Check sheet for the modelled part. Datum: model origin and axes. Units: mm. A direction names the side the tool comes from. Round coordinates to 2 decimals unless told otherwise and drop trailing zeros. Order: outer loops, then holes, each group sorted by start corner. A loop starts at its lowest first (then second) coordinate and runs counter-clockwise, first axis right, second up. Notation, with made-up numbers: M 49,47 L 68,47 A21 ccw 68,60 Z; hole C 76,50.5 d4. An arc over 180 degrees is marked long. One line per item, written item: value. Start each with the question number.
(1) Access from +Z, -Z, +X, -X, +Y, -Y to the whole of each face (thin tool, end or side, straight path). Record for faces 1 (the face through (6.35, 2, 13)), 2 (the face through (27.49, 1.57, -8.02)), 3 (the face through (15.89, 1.57, -23.79)).
(2) Cross-section at A-A, the plane x = 11. Enter the section's corners in (y, z) (3 decimals).
(3) Cross-section at C-C, the plane y = 0.6. Count the separate pieces of the cut face and the enclosed holes in it, and give its area (3 significant figures).
(4) Depth check by flat-ended pin: pin 1 Ø1.5 at (y, z) = (0.5, -19) entering from -X; pin 2 Ø1.6 at (y, z) = (2, 14.5) entering from +X. Enter the tip coordinate at first touch or a pass-through.
(5) Release check for a two-part mould opening along X. For faces 4 (the face through (17.342, 1.565, 22.794)), 5 (the face through (28.44, 1.57, 3.36)), 6 (the face through (0, 2, 17)) record: released by +X, released by -X, zero draft, split by the parting line, or undercut.
(6) Thickness scan on L1, parallel to Z at x = 27.5, y = 1.3; L2, parallel to X at y = 2.9, z = 8.5; L3, parallel to Z at x = 6.5, y = 1. Record the ranges inside material, lowest first.
from build123d import *

# Parameters (mm, degrees)
BOSS_EXTRUDE1_DEPTH = 3.175
CUT_EXTRUDE1_DEPTH  = 3.175
CIRPATTERN1_DEPTH   = 3.175
SKETCH3_R           = 1
CUT_EXTRUDE2_DEPTH  = 3.175


# Read off the part's stored shape, not the designer's step: CirPattern1
with BuildPart() as part:
    # Sketch1 → Boss-Extrude1 (new body)
    with BuildSketch(Plane(origin=(0, 0, 0), x_dir=(1, 0, 0), z_dir=(0, 1, 0))):
        with BuildLine():
            Line((0, 29.6545), (0, 6.35))
            ThreePointArc((0, 6.35), (-6.35, 0), (0, -6.35))
            Line((0, -6.35), (0, -29.6545))
            ThreePointArc((0, -29.6545), (29.6545, 0), (0, 29.6545))
        make_face()
        with BuildLine():
            Line((6.35, 22.422694313), (6.35, 3.666174209))
            Line((6.35, 3.666174209), (20.182289022, 11.65225))
            ThreePointArc((20.182289022, 11.65225), (14.317514025, 18.387727222), (6.35, 22.422694313))
        make_face(mode=Mode.SUBTRACT)
        with BuildLine():
            Line((6.35, 0), (21.581607168, -8.793972499))
            ThreePointArc((21.581607168, -8.793972499), (23.3045, 0), (21.581607168, 8.793972499))
            Line((21.581607168, 8.793972499), (6.35, 0))
        make_face(mode=Mode.SUBTRACT)
        with BuildLine():
            Line((6.35, -3.666174209), (20.182289022, -11.65225))
            ThreePointArc((20.182289022, -11.65225), (14.317514025, -18.387727222), (6.35, -22.422694313))
            Line((6.35, -22.422694313), (6.35, -3.666174209))
        make_face(mode=Mode.SUBTRACT)
    extrude(amount=BOSS_EXTRUDE1_DEPTH)

    # Sketch2 → Cut-Extrude1 (cut)
    with BuildSketch(Plane(origin=(0, 3.175, 0), x_dir=(1, 0, 0), z_dir=(0, 1, 0))):
        Polygon((2.009170374, 29.586358422), (2.730257833, 27.469749607), (4.711979869, 27.199976048), (5.972614446, 29.046811304), align=None)
    extrude(amount=-CUT_EXTRUDE1_DEPTH, mode=Mode.SUBTRACT)


with BuildPart() as body_2:
    # of the pieces the cut leaves, the one that is kept (cut_extrude1_keep)
    add(part.part.solids().sort_by_distance((0, 0, -29.6545))[0])

    # CirPattern1 outline → CirPattern1 (cut)
    with BuildSketch(Plane(origin=(0, 0, 0), x_dir=(1, 0, 0), z_dir=(0, 1, 0))):
        with BuildLine():
            ThreePointArc((11.643715218, 27.272940182), (9.777824138, 27.996134115), (7.867406851, 28.59183939))
            Line((7.867406851, 28.59183939), (8.152034339, 26.373960405))
            Line((8.152034339, 26.373960405), (10.040188522, 25.714510801))
            Line((10.040188522, 25.714510801), (11.643715218, 27.272940182))
        make_face()
        with BuildLine():
            ThreePointArc((0, -29.6545), (0.935371957, -29.639744425), (1.869813063, -29.595492382))
            Line((1.869813063, -29.595492382), (0.878621718, -27.591112249))
            Line((0.878621718, -27.591112249), (0, -27.587246726))
            Line((0, -27.587246726), (0, -29.6545))
        make_face()
        with BuildLine():
            ThreePointArc((3.809498846, -29.408792712), (5.784253675, -29.084906389), (7.732668198, -28.628573363))
            Line((7.732668198, -28.628573363), (6.361766185, -26.862043524))
            Line((6.361766185, -26.862043524), (4.400181509, -27.252153199))
            Line((4.400181509, -27.252153199), (3.809498846, -29.408792712))
        make_face()
        with BuildLine():
            ThreePointArc((9.596192288, -28.058910596), (11.466730783, -27.347823595), (13.285052137, -26.51220021))
            Line((13.285052137, -26.51220021), (11.589481982, -25.054447882))
            Line((11.589481982, -25.054447882), (9.745052057, -25.827803075))
            Line((9.745052057, -25.827803075), (9.596192288, -28.058910596))
        make_face()
        with BuildLine():
            ThreePointArc((14.997592941, -25.582446643), (16.688811877, -24.512709528), (18.304033384, -23.331346556))
            Line((18.304033384, -23.331346556), (16.35187323, -22.240901357))
            Line((16.35187323, -22.240901357), (14.698653008, -23.3664514))
            Line((14.698653008, -23.3664514), (14.997592941, -25.582446643))
        make_face()
        with BuildLine():
            ThreePointArc((19.796831377, -22.078832344), (21.240827314, -20.693395692), (22.588096877, -19.213725556))
            Line((22.588096877, -19.213725556), (20.457727108, -18.534369503))
            Line((20.457727108, -18.534369503), (19.062094358, -19.966922897))
            Line((19.062094358, -19.966922897), (19.796831377, -22.078832344))
        make_face()
        with BuildLine():
            ThreePointArc((23.801215338, -17.688739883), (24.940010987, -16.043229793), (25.965234936, -14.324662123))
            Line((25.965234936, -14.324662123), (23.742191157, -14.083671764))
            Line((23.742191157, -14.083671764), (22.660181358, -15.765710644))
            Line((22.660181358, -15.765710644), (23.801215338, -17.688739883))
        make_face()
        with BuildLine():
            ThreePointArc((26.849966443, -12.588434067), (27.637838485, -10.748918742), (28.299853474, -8.860455044))
            Line((28.299853474, -8.860455044), (26.073392205, -9.067506284))
            Line((26.073392205, -9.067506284), (25.348448689, -10.931495795))
            Line((25.348448689, -10.931495795), (26.849966443, -12.588434067))
        make_face()
        with BuildLine():
            ThreePointArc((28.820675533, -6.982695186), (29.22599044, -5.023032253), (29.498216176, -3.04049546))
            Line((29.498216176, -3.04049546), (27.357731153, -3.68727507))
            Line((27.357731153, -3.68727507), (27.018960831, -5.658374932))
            Line((27.018960831, -5.658374932), (28.820675533, -6.982695186))
        make_face()
        with BuildLine():
            ThreePointArc((29.634217474, -1.096596968), (29.640701614, 0.904531949), (29.512208073, 2.901541813))
            Line((29.512208073, 2.901541813), (27.543641034, 1.841002417))
            Line((27.543641034, 1.841002417), (27.604645734, -0.158066973))
            Line((27.604645734, -0.158066973), (29.634217474, -1.096596968))
        make_face()
        with BuildLine():
            ThreePointArc((29.257928078, 4.833530266), (28.865321108, 6.795778658), (28.341267381, 8.727080467))
            Line((28.341267381, 8.727080467), (26.623657455, 7.295362569))
            Line((26.623657455, 7.295362569), (27.081987803, 5.348587468))
            Line((27.081987803, 5.348587468), (29.257928078, 4.833530266))
        make_face()
        with BuildLine():
            ThreePointArc((27.706915584, 10.569588405), (26.930980906, 12.41417084), (26.03240806, 14.202221686))
            Line((26.03240806, 14.202221686), (24.634718301, 12.456809604))
            Line((24.634718301, 12.456809604), (25.471972063, 10.640492963))
            Line((25.471972063, 10.640492963), (27.706915584, 10.569588405))
        make_face()
        with BuildLine():
            ThreePointArc((25.043454062, 15.881271325), (23.915345912, 17.534126729), (22.678332178, 19.107135313))
            Line((22.678332178, 19.107135313), (21.656680655, 17.118108374))
            Line((21.656680655, 17.118108374), (22.839241597, 15.50517638))
            Line((22.839241597, 15.50517638), (25.043454062, 15.881271325))
        make_face()
        with BuildLine():
            ThreePointArc((21.374483065, 20.555311819), (19.939495651, 21.950077071), (18.413707861, 23.24488617))
            Line((18.413707861, 23.24488617), (17.809114486, 21.092104981))
            Line((17.809114486, 21.092104981), (19.289502088, 19.747317805))
            Line((19.289502088, 19.747317805), (21.374483065, 20.555311819))
        make_face()
        with BuildLine():
            ThreePointArc((16.847313945, 24.4040444), (15.16306286, 25.484718851), (13.409762295, 26.449341116))
            Line((13.409762295, 26.449341116), (13.24650185, 24.219241112))
            Line((13.24650185, 24.219241112), (14.965277675, 23.196592754))
            Line((14.965277675, 23.196592754), (16.847313945, 24.4040444))
        make_face()
    extrude(amount=CIRPATTERN1_DEPTH, mode=Mode.SUBTRACT)

    # Sketch3 → Cut-Extrude2 (cut)
    with BuildSketch(Plane(origin=(0, 3.175, 0), x_dir=(1, 0, 0), z_dir=(0, 1, 0))):
        with Locations(Location((0, 0, 0), (0, 0, 270))):
            Circle(SKETCH3_R)
    extrude(amount=-CUT_EXTRUDE2_DEPTH, mode=Mode.SUBTRACT)


solid = body_2.part
Values found:
1. face 1: +Y, -Y
1. face 2: +X, +Y, -Y
1. face 3: -Z, +Y, -Y
2. outline: M 0,-26.647 L 3.175,-26.647 L 3.175,-20.545 L 0,-20.545 Z; M 0,-6.351 L 3.175,-6.351 L 3.175,-2.685 L 0,-2.685 Z; M 0,2.685 L 3.175,2.685 L 3.175,6.351 L 0,6.351 Z; M 0,20.545 L 3.175,20.545 L 3.175,25.302 L 0,25.302 Z
3. separate pieces: 1
3. enclosed holes: 4
3. area: 892 mm^2
4. pin 1: x = 0
4. pin 2: x = 26.3
5. face 4: undercut
5. face 5: released by +X
5. face 6: released by -X
6. L1: -10.58 to -8.03, -5.25 to 3.64, 6.01 to 8.93
6. L2: 0 to 6.35, 14.72 to 21.07, 21.7 to 28.41
6. L3: -28.93 to -22.38, -3.75 to -0.09, 0.09 to 3.75, 22.38 to 27.04
